Read the model definition and answer for the solid it produces. Units are mm, in the model's axes. Give positions to 0.01 mm unless a question says otherwise; leave off trailing zeros. Write each loop counter-clockwise with the first axis right and the second up, starting at its lowest first coordinate (ties: lowest second). Pieces come first, ordered by that corner, then holes. Notation, with made-up numbers: M 44.25,-36 L 53.25,-36 A19 ccw 53.25,-4 Z; hole C -31,38.5 d1. An arc over 180 degrees is marked long. Put each result on its own line as item: value.
from build123d import *

# Parameters (mm, degrees)
F0_W     = 146.05
F0_H     = 76.2
F0_W_2   = 12.7
F0_H_2   = 63.5
F0_R     = 25.4
F1_DEPTH = 1.5875


with BuildPart() as f1:
    # F0 (on Front) → F1 (new body, symmetric)
    with BuildSketch(Plane.XZ):
        Rectangle(F0_W, F0_H)
        with Locations((-61.460756, 0)):
            Rectangle(F0_W_2, F0_H_2, mode=Mode.SUBTRACT)
        Circle(F0_R, mode=Mode.SUBTRACT)
    extrude(amount=F1_DEPTH, both=True)


solid = f1.part
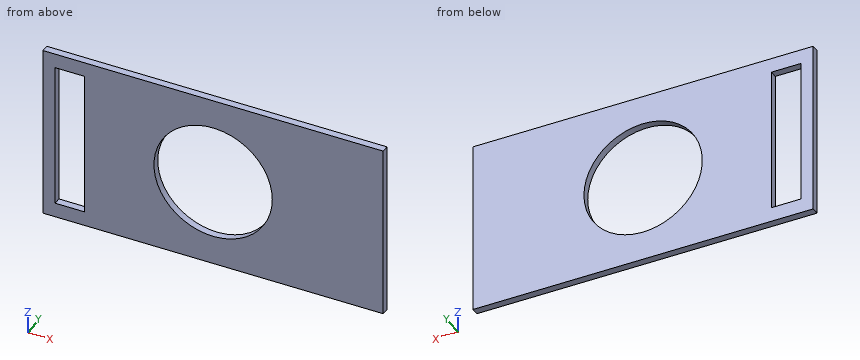
(1) Section B-B on x = 0 is taken. Determine the outline of the cut face in (y, z), and give its area (3 significant figures).
Result:
outline: M -1.59,-38.1 L 1.59,-38.1 L 1.59,-25.4 L -1.59,-25.4 Z; M -1.59,25.4 L 1.59,25.4 L 1.59,38.1 L -1.59,38.1 Z
area: 80.6 mm²
(2) Section D-D on z = -27 is taken. Determine the outline of the cut face in (x, y) (1 decimal).
Result:
outline: M -73,-1.6 L -67.8,-1.6 L -67.8,1.6 L -73,1.6 Z; M -55.1,-1.6 L 73,-1.6 L 73,1.6 L -55.1,1.6 Z
(3) Section C-C on y = 1 is taken. Determine the outline of the cut face in (x, z) (3 decimals).
Result:
outline: M -73.025,-38.1 L 73.025,-38.1 L 73.025,38.1 L -73.025,38.1 Z; hole M -67.811,-31.75 L -55.111,-31.75 L -55.111,31.75 L -67.811,31.75 Z; hole C 0,0 d50.8
(4) Straight lines are drawn through the part: line 1 along Z through (x, y) = (-57.5, -1.4); line 2 along X through (y, z) = (-0.7, 1.5) (3 decimals); line 3 along X through (y, z) = (-1.1, 13) (3 decimals). For each, find the intervals that lie inside material, in ascending order. Write a range as from..to.
Result:
line 1: z = -38.1..-31.75, 31.75..38.1
line 2: x = -73.025..-67.811, -55.111..-25.356, 25.356..73.025
line 3: x = -73.025..-67.811, -55.111..-21.821, 21.821..73.025
(5) Section A-A on z = 0 is taken. Determine the outline of the cut face in (x, y) (1 decimal), and give its area (3 significant figures).
Result:
outline: M -73,-1.6 L -67.8,-1.6 L -67.8,1.6 L -73,1.6 Z; M -55.1,-1.6 L -25.4,-1.6 L -25.4,1.6 L -55.1,1.6 Z; M 25.4,-1.6 L 73,-1.6 L 73,1.6 L 25.4,1.6 Z
area: 262 mm²
